from build123d import *

# Parameters (mm, degrees)
SKETCH1_W                  = 539
SKETCH1_H                  = 299
BOSS_EXTRUDE1_DEPTH        = 5
SKETCH5_W                  = 70
SKETCH5_H                  = 20
CUT_EXTRUDE2_DEPTH         = 309.229622197
SKETCH2_W                  = 30
SKETCH2_H                  = 51
CUT_EXTRUDE1_DEPTH         = 309.229622197
F_5_5_5_5_DIAMETER_HOLE1_D = 5.5
LPATTERN1_COUNT            = 7
LPATTERN1_PITCH            = 85
LPATTERN1_COUNT_DIR2       = 4
LPATTERN1_PITCH_DIR2       = 70
FILLET1_R                  = 0.5


with BuildPart() as part:
    # Sketch1 → Boss-Extrude1 (new body)
    with BuildSketch(Plane(origin=(0, 0, 0), x_dir=(1, 0, 0), z_dir=(0, 1, 0))):
        Rectangle(SKETCH1_W, SKETCH1_H)
    extrude(amount=BOSS_EXTRUDE1_DEPTH)

    # Sketch5 → Cut-Extrude2 (cut, through all)
    with BuildSketch(Plane(origin=(0, 5, 0), x_dir=(1, 0, 0), z_dir=(0, 1, 0))):
        Polygon((269.5, 149.5), (199.5, 149.5), (199.5, 129.5), (249.5, 129.5), (249.5, 91.5), (269.5, 91.5), align=None)
        with Locations((234.5, -139.5)):
            Rectangle(SKETCH5_W, SKETCH5_H)
    extrude(amount=-CUT_EXTRUDE2_DEPTH, mode=Mode.SUBTRACT)

    # Sketch2 → Cut-Extrude1 (cut, through all)
    with BuildSketch(Plane(origin=(0, 5, 0), x_dir=(1, 0, 0), z_dir=(0, 1, 0))):
        with Locations((-254.5, 0)):
            Rectangle(SKETCH2_W, SKETCH2_H)
    cut_extrude1 = extrude(amount=-CUT_EXTRUDE1_DEPTH, mode=Mode.SUBTRACT)

    # Mirror1: Cut-Extrude1 across plane
    add(cut_extrude1.mirror(Plane(origin=(0, 0, 0), x_dir=(0, 0, 1), z_dir=(1, 0, 0))), mode=Mode.SUBTRACT)

    # Ø5.5 (5.5) Diameter Hole1 (through all)
    with Locations(Plane(origin=(-255, 5, 105), x_dir=(0, 0, 1), z_dir=(0, 1, 0))):
        with Locations((0, 0)):
            f_5_5_5_5_diameter_hole1 = Hole(F_5_5_5_5_DIAMETER_HOLE1_D / 2)

    # LPattern1: 5.5 _5.5_ Diameter Hole1 7 × 4, 1 skipped
    with Locations(*[(i * LPATTERN1_PITCH, 0, -j * LPATTERN1_PITCH_DIR2) for i in range(LPATTERN1_COUNT) for j in range(LPATTERN1_COUNT_DIR2) if (i, j) not in ((0, 0), (6, 3))]):
        add(f_5_5_5_5_diameter_hole1, mode=Mode.SUBTRACT)

    # Fillet1
    fillet1_edges = [part.edges().sort_by_distance(p)[0] for p in [
        (269.5, 2.5, -91.5),
        (249.5, 2.5, -91.5),
        (249.5, 2.5, -129.5),
        (199.5, 2.5, -129.5),
        (199.5, 2.5, -149.5),
        (269.5, 2.5, 129.5),
        (199.5, 2.5, 149.5),
        (199.5, 2.5, 129.5),
        (-269.5, 2.5, 25.5),
        (-269.5, 2.5, -25.5),
        (-239.5, 2.5, -25.5),
        (-239.5, 2.5, 25.5),
        (269.5, 2.5, -25.5),
        (269.5, 2.5, 25.5),
        (239.5, 2.5, 25.5),
        (239.5, 2.5, -25.5),
        (-269.5, 2.5, -149.5),
        (-269.5, 2.5, 149.5),
    ]]
    fillet(fillet1_edges, radius=FILLET1_R)


solid = part.part
The model under review builds one solid part; all positions refer to its coordinate system, in mm. Give positions to 0.01 mm unless a question says otherwise; leave off trailing zeros. Write each loop counter-clockwise with the first axis right and the second up, starting at its lowest first coordinate (ties: lowest second). Pieces come first, ordered by that corner, then holes.
1. Wall thickness on L1, parallel to Z at x = -241, y = 4.2; L2, parallel to Z at x = 226.5, y = 3.7; L3, parallel to X at y = 1.3, z = 24.5: over which ranges is each line inside the solid? List them lowest first.
2. Add section C-C, the plane z = -12.5. Write out the cut boundary in (x, y), plus the area to 4 significant figures.
3. Add section A-A, the plane y = 2.35. Count the separate pieces of the cut face and the enclosed holes in it, plus the area to 3 significant figures.
4. Add section B-B, the plane x = 218. Write out the cut boundary in (y, z).
5. For P1, Ø5, axis at x = 85, z = 35, coming from the -Y side; P2, Ø1.5, axis at y = 1.5, z = 137, coming from the +X side, all flat-tipped, find the tip position at first contact; note any pin that passes through.
Worked answers:
1. L1: z = -149.5 to -25.5, 25.5 to 149.5
1. L2: z = -129.5 to 129.5
1. L3: x = -239.5 to 239.5
2. outline: (-239.5, 0) - (239.5, 0) - (239.5, 5) - (-239.5, 5) - close
2. area: 2,395 mm2
3. separate pieces: 1
3. enclosed holes: 27
3. area: 154,000 mm2
4. outline: (0, -129.5) - (5, -129.5) - (5, 129.5) - (0, 129.5) - close
5. P1: passes through
5. P2: stops at x = 199.5
